Input: part model. Units: mm. Frame: model coordinates. A direction names the side the tool comes from. Round coordinates to 2 decimals unless told otherwise and drop trailing zeros. Loops run counter-clockwise (first coordinate to the right, second up) from the corner with the lowest first, then second, coordinate; pieces in that order, holes last.
1) Draft query along Y for faces 5 (the face through (-9.906, 19, 0)), 6 (the face through (0, -15.24, 0)), 7 (the face through (3.112, 0, 0)). Return one class per face: pulls with the +Y half, pulls with the -Y half, needs draft (parallel to the pull), parting line crosses it, or undercut.
2) Ray query, line 1 along X through (y, z) = (-1, 0.75); line 2 along Z through (x, y) = (-4, -16); line 3 along Y through (x, z) = (3, -3.5). Return the intervals inside material, ascending.
3) Section D-D, the plane y = 11. Return loops of the section in (x, z), and give its area (3 significant figures).
4) First-contact query: pin 1 (1 mm diameter, centred on x = 0, z = 0.5, fed in from -Y); pin 2 (1.3 mm diameter, centred on x = 16.5, z = -0.5, fed in from +Y); pin 3 (3 mm diameter, centred on y = 19.5, z = -1, fed in from -X). Flat tips, straight axial feed; report the tip coordinate or a pass-through.
5) Section A-A, the plane y = -9. Return loops of the section in (x, z), and give its area (3 significant figures).
6) Section C-C, the plane x = -5.5. Return loops of the section in (y, z).
7) Access query for faces 1 (the face through (17, 10.16, 0)), 2 (the face through (0, 19, -2.286)), 3 (the face through (-19, -9.906, 0)), 4 (the face through (0, -12.7, 0)). Directions: +Z, -Z, +X, -X, +Y, -Y. A direction counts if a zero-diameter tool reaches every point of the face in a straight line with its end or side. Return the directions, or none.
8) Section B-B, the plane z = 0.25. Return loops of the section in (x, y).
from build123d import *

# Parameters (mm, degrees)
F0_W     = 35.56
F0_H     = 35.56
F0_W_2   = 5.3412760417
F0_H_2   = 25.1850260417
F1_DEPTH = 5.08
F2_W     = 19.812
F2_H     = 4.572
F3_DEPTH = 2.54
F4_W     = 19.812
F4_H     = 4.572
F5_DEPTH = 2.54
F6_W     = 20.32
F6_H     = 5.08
F7_DEPTH = 2.54
F8_W     = 20.32
F8_H     = 5.08
F9_DEPTH = 2.54


with BuildPart() as f1:
    # F0 (on Top) → F1 (new body, symmetric)
    with BuildSketch(Plane.XY):
        Rectangle(F0_W, F0_H)
        with Locations((0.4409722222, -0.1074869792)):
            Rectangle(F0_W_2, F0_H_2, mode=Mode.SUBTRACT)
    extrude(amount=F1_DEPTH, both=True)

    # F2 (on face) → F3 (join)
    with BuildSketch(Plane(origin=(0, 17.78, 0), x_dir=(-1, 0, 0), z_dir=(0, 1, 0))):
        Rectangle(F2_W, F2_H)
    extrude(amount=F3_DEPTH)

    # F4 (on face) → F5 (join)
    with BuildSketch(Plane(origin=(-17.78, 0, 0), x_dir=(0, -1, 0), z_dir=(-1, 0, 0))):
        Rectangle(F4_W, F4_H)
    extrude(amount=F5_DEPTH)

    # F6 (on face) → F7 (cut)
    with BuildSketch(Plane.XZ.offset(17.78)):
        Rectangle(F6_W, F6_H)
    extrude(amount=-F7_DEPTH, mode=Mode.SUBTRACT)

    # F8 (on face) → F9 (cut)
    with BuildSketch(Plane.YZ.offset(17.78)):
        Rectangle(F8_W, F8_H)
    extrude(amount=-F9_DEPTH, mode=Mode.SUBTRACT)


solid = f1.part
Final values:
1. face 5: needs draft
1. face 6: pulls with the -Y half
1. face 7: undercut
2. line 1: x = -20.32 to -2.23, 3.11 to 15.24
2. line 2: z = -5.08 to -2.54, 2.54 to 5.08
2. line 3: y = -17.78 to -12.7, 12.49 to 17.78
3. outline: (-17.78, -5.08) - (-2.23, -5.08) - (-2.23, 5.08) - (-17.78, 5.08) - close; (3.11, -5.08) - (17.78, -5.08) - (17.78, 5.08) - (3.11, 5.08) - close
3. area: 307 mm2
4. pin 1: stops at y = -15.24
4. pin 2: stops at y = 17.78
4. pin 3: stops at x = -9.91
5. outline: (-20.32, -2.29) - (-17.78, -2.29) - (-17.78, -5.08) - (-2.23, -5.08) - (-2.23, 5.08) - (-17.78, 5.08) - (-17.78, 2.29) - (-20.32, 2.29) - close; (3.11, -5.08) - (17.78, -5.08) - (17.78, -2.54) - (15.24, -2.54) - (15.24, 2.54) - (17.78, 2.54) - (17.78, 5.08) - (3.11, 5.08) - close
5. area: 306 mm2
6. outline: (-17.78, -5.08) - (17.78, -5.08) - (17.78, -2.29) - (20.32, -2.29) - (20.32, 2.29) - (17.78, 2.29) - (17.78, 5.08) - (-17.78, 5.08) - (-17.78, 2.54) - (-15.24, 2.54) - (-15.24, -2.54) - (-17.78, -2.54) - close
7. face 1: +X
7. face 2: -Z, +X, -X, +Y
7. face 3: +Z, -Z, -X, -Y
7. face 4: +Z, -Z
8. outline: (-20.32, -9.91) - (-17.78, -9.91) - (-17.78, -17.78) - (-10.16, -17.78) - (-10.16, -15.24) - (10.16, -15.24) - (10.16, -17.78) - (17.78, -17.78) - (17.78, -10.16) - (15.24, -10.16) - (15.24, 10.16) - (17.78, 10.16) - (17.78, 17.78) - (9.91, 17.78) - (9.91, 20.32) - (-9.91, 20.32) - (-9.91, 17.78) - (-17.78, 17.78) - (-17.78, 9.91) - (-20.32, 9.91) - close; hole (-2.23, -12.7) - (3.11, -12.7) - (3.11, 12.49) - (-2.23, 12.49) - close
